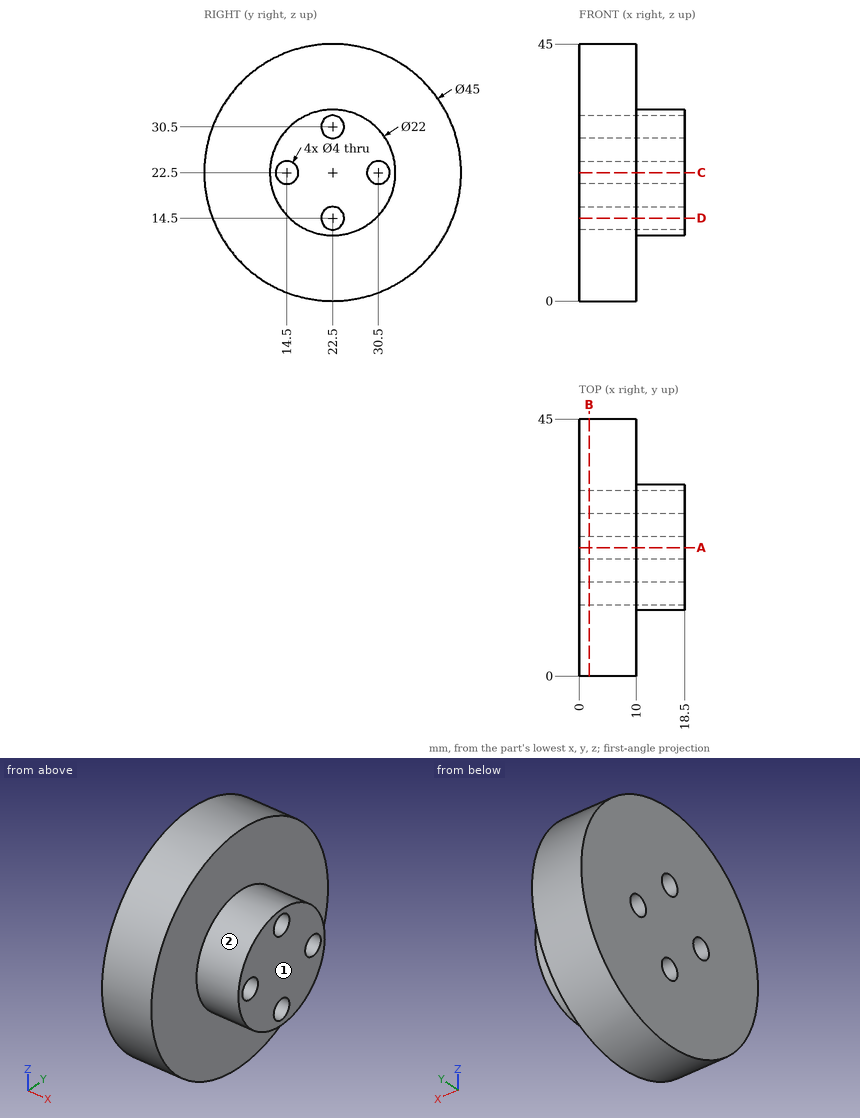
Check sheet for the drawn part. Datum: minimum x, y, z corner. Units: mm. A direction names the side the tool comes from. Round coordinates to 2 decimals unless told otherwise and drop trailing zeros. Loops run counter-clockwise (first coordinate to the right, second up) from the corner with the lowest first, then second, coordinate; pieces in that order, holes last. Notation, with made-up numbers: (-5.5, 80) - (39.5, 80) arc R17 cw to (39.5, 85) - close; hole circle Ø1 at (-19.5, 17.5). An arc over 180 degrees is marked (long way). Write each question's results on one line, items separated by ' | '. Start each with the question number.
Q1. Cross-section at D-D on z = 14.5. Enter the section's corners in (x, y), and give its area (3 significant figures).
Q2. Gauge pin test, flat ends, axial feed: P1, Ø1.5, axis at x = 10.5, y = 26.5, coming from the +Z side; P2, Ø4, axis at x = 10, y = 10, coming from the -Z side; P3, Ø2, axis at x = 3.5, y = 35.5, coming from the +Z side. Record the tip position at first contact, or that the pin passes through.
Q3. Cross-section at B-B on x = 1.75. Enter the section's corners in (y, z), and give its area (3 significant figures).
Q4. Access from +Z, -Z, +X, -X, +Y, -Y to the whole of each face (thin tool, end or side, straight path). Record for the marked faces 1 and 2.
Q5. Thickness scan on line 1 (Y direction, x = 4.25, z = 22.5); line 2 (Y direction, x = 13, z = 22.5); line 3 (X direction, y = 26, z = 36). Record the ranges inside material, lowest first. Write a range as [from, to].
Q6. Cross-section at A-A on y = 22.5. Enter the section's corners in (x, z), and give its area (3 significant figures).
Answers below:
1) outline: (0, 1.47) - (10, 1.47) - (10, 14.95) - (18.5, 14.95) - (18.5, 20.5) - (0, 20.5) - close; (0, 24.5) - (18.5, 24.5) - (18.5, 30.05) - (10, 30.05) - (10, 43.53) - (0, 43.53) - close | area: 475 mm²
2) P1: stops at z = 44.74 | P2: stops at z = 2.6 | P3: stops at z = 41.53
3) outline: circle Ø45 at (22.5, 22.5); hole circle Ø4 at (14.5, 22.5); hole circle Ø4 at (22.5, 14.5); hole circle Ø4 at (22.5, 30.5); hole circle Ø4 at (30.5, 22.5) | area: 1,540 mm²
4) face 1: +Z, -Z, +X, +Y, -Y | face 2: +X
5) line 1: y = [0, 12.5], [16.5, 28.5], [32.5, 45] | line 2: y = [11.5, 12.5], [16.5, 28.5], [32.5, 33.5] | line 3: x = [0, 10]
6) outline: (0, 0) - (10, 0) - (10, 11.5) - (18.5, 11.5) - (18.5, 12.5) - (0, 12.5) - close; (0, 16.5) - (18.5, 16.5) - (18.5, 28.5) - (0, 28.5) - close; (0, 32.5) - (18.5, 32.5) - (18.5, 33.5) - (10, 33.5) - (10, 45) - (0, 45) - close | area: 489 mm²
